Autodesk Inventor part; units mm, degrees
ref_plane "YZ Plane" through (0, 0, 0) normal (1, 0, 0) x (0, 1, 0)
ref_plane "XZ Plane" through (0, 0, 0) normal (0, 1, 0) x (-1, 0, 0)
ref_plane "XY Plane" through (0, 0, 0) normal (0, 0, 1) x (1, 0, 0)
sketch "Эскиз1" plane through (0, 0, 0) normal (0, 0, 1) x (1, 0, 0)
  line L0 (-19.4221, 3.2482) -> (-17.0252, 13.9839)
  line L1 (17.0252, 13.9839) -> (19.4221, 3.2482)
  arc A0 (-41.5809, 15.0397) -> (41.5809, 15.0397) centre (0, 65) ccw
  line L2 (41.5809, 15.0397) -> (33.2647, 25.0318)
  arc A1 (-33.2647, 25.0318) -> (33.2647, 25.0318) centre (0, 65) ccw
  line L3 (-33.2647, 25.0318) -> (-41.5809, 15.0397)
  line L4 (-5.5, 11.5) -> (-5.5, 0.5)
  line L5 (5.5, 0.5) -> (5.5, 11.5)
  circle A2 centre (0, 65) radius 65
  circle A3 centre (0, 65) radius 52
  line L6 (-41.5809, 15.0397) -> (-33.2647, 25.0318)
  line L7 (20.5764, 3.3428) -> (0, 65)
  line L8 (-41.5809, 15.0397) -> (0, 65)
  line L9 (0, 65) -> (21.1137, 3.5247)
  line L10 (-32.5, 8.7083) -> (0, 65)
  line L11 (0, 65) -> (32.5, 8.7083)
  line L12 (0, 65) -> (0, 0)
  arc A4 (-39.7976, 13.9446) -> (-45.7382, 14.0977) centre (-42.8715, 10.0011) ccw
  line L13 (-45.7382, 14.0977) -> (-66.813, -0.6503)
  line L14 (-66.813, -0.6503) -> (-66.8135, -2.4814)
  line L15 (-66.8135, -2.4814) -> (-61.8135, -2.4828)
  line L16 (-61.8135, -2.4828) -> (-61.8127, 0.4976)
  arc A5 (-61.386, 1.3167) -> (-61.8127, 0.4976) centre (-60.8127, 0.4974) ccw
  line L17 (-61.386, 1.3167) -> (-46.2094, 11.9372)
  arc A6 (-40.3216, 11.8247) -> (-46.2094, 11.9372) centre (-43.3426, 7.8406) ccw
  arc A7 (-40.3216, 11.8247) -> (-21.0718, 1.6801) centre (0, 65) ccw
  line L18 (-21.0718, 1.6801) -> (-20.6332, 3.6423)
  arc A8 (-39.7976, 13.9446) -> (-20.6332, 3.6423) centre (0, 65) ccw
  circle A9 centre (0, 65) radius 64.7341
  arc A10 (-42.6225, 16.2781) -> (-20.6332, 3.6423) centre (0, 65) ccw
  line L19 (-42.6225, 16.2781) -> (0, 65)
  point P0 (0, 0)
  point P1 (0, 13)
  point P2 (-26, 19.9667)
  point P3 (-32.5, 8.7083)
  point P4 (32.5, 8.7083)
  point P5 (26, 19.9667)
  dimension "d23" = 0.5
  dimension "d25" = 60
  dimension "d26" = 30
  dimension "d42" = 60.135
extrude "Выдавливание1" add sketch "Эскиз1" along normal blind 10 contours L7 A9 L1 | L7 A1 L9 A9 | L1 A9 L12 A1 L7 | A9 L7 A0 L12 | A9 L9 A0 L7 | A9 L11 A0 L9 | L9 A1 L11 A9 | L12 A9 A8 L10 A1 | L12 A0 L18 A9 | A0 L10 A8 L18
sketch "Эскиз4" plane through (0, 0, 10) normal (0, 0, 1) x (1, 0, 0)
  arc A0 (-13.3607, 13.1952) -> (-9.9415, 12.4318) centre (0, 65) ccw
  circle A1 centre (0, 65) radius 53.5
  circle A2 centre (0, 65) radius 54.5
  line L0 (-26, 19.9667) -> (-32.5, 8.7083)
  arc A3 (-26, 19.9667) -> (-22.4589, 18.1001) centre (0, 65) ccw
  arc A4 (-26, 19.9667) -> (26, 19.9667) centre (0, 65) ccw
  arc A5 (22.4589, 18.1001) -> (26, 19.9667) centre (0, 65) ccw
  line L1 (32.5, 8.7083) -> (26, 19.9667)
  point P0 (0, 0)
  point P1 (-27.25, 17.8016)
  point P2 (27.25, 17.8016)
  dimension "d43" = 1
extrude "Выдавливание4" cut sketch "Эскиз4" against normal blind 5 contours A1 L0 A3 A4 L1 A0 | A0 A1 L1 A2 L0
draft "НаклГрань1" angle 10 pull direction (0, 0, -1) faces at (-30.75, 11.7394, 5) fixed edges at (-26.625, 18.8841, 5)
draft "НаклГрань2" angle 10 pull direction (0, 0, -1) faces at (30.75, 11.7394, 5) fixed edges at (26.625, 18.8841, 5)
sketch "Эскиз5" plane through (0, 0, 10) normal (0, 0, 1) x (1, 0, 0)
  arc A0 (-26, 19.9667) -> (26, 19.9667) centre (0, 65) ccw
  line L0 (-27.25, 17.8016) -> (-26, 19.9667)
  arc A1 (-27.25, 17.8016) -> (27.25, 17.8016) centre (0, 65) ccw
  line L1 (26, 19.9667) -> (27.25, 17.8016)
  point P0 (0, 0)
extrude "Выдавливание5" cut sketch "Эскиз5" against normal blind 6
sketch "Эскиз6" plane through (0, 0, 0) normal (0, 0, -1) x (-1, 0, 0)
  line L0 (-31.7335, 8.2727) -> (-25.2327, 19.5323)
  arc A0 (-25.2327, 19.5323) -> (25.2327, 19.5323) centre (0, 65) ccw
  arc A1 (-31.7335, 8.2727) -> (31.7335, 8.2727) centre (0, 65) ccw
  line L1 (25.2327, 19.5323) -> (31.7335, 8.2727)
  circle A2 centre (0, 20) radius 1.925
  circle A3 centre (0, 20) radius 4
  circle A4 centre (0, 20) radius 1.6
  circle A5 centre (0, 20) radius 4
  line L2 (-2.8284, 22.8284) -> (-11.3933, 14.2635)
  line L3 (2.8284, 22.8284) -> (11.3933, 14.2635)
  line L4 (0, 89.6007) -> (0, 9.3033)
  point P0 (0, 0)
  dimension "d50" = 3.2
  dimension "d51" = 8
  dimension "d52" = 45
  dimension "d53" = 45
extrude "Выдавливание6" add sketch "Эскиз6" against normal blind 2.5 contours L2 A3 L4 A0 | L4 A3 L3 A0 | A3 L4 A2 | L4 A2 A3 | L4 A4 A2 | A2 L4 A4
equation "\"d26\" = 0.5 * d25"
properties part number "vzuh_karetka"
Geometry: final body of the model. Coordinates: model frame, mm. A direction names the side the tool comes from. Round coordinates to 2 decimals unless told otherwise and drop trailing zeros. Order: outer loops, then holes, each group sorted by start corner. A loop starts at its lowest first (then second) coordinate and runs counter-clockwise, first axis right, second up. Notation, with made-up numbers: M 31,-33 L 65,-33 A31 cw 65,-7 Z; hole C -16.5,3 d5. An arc over 180 degrees is marked long. Use one line per item in the form item = value. Start each with the question number.
Q1. Cut plane B-B (z = 1.5). Return loops of the section in (x, y).
Q2. Material intervals for line 1 (Y direction, x = 0, z = 1.55); line 2 (Z direction, x = 2, y = 12); line 3 (Z direction, x = -6, y = 18.75), sorted ascending. Write a range as [from, to].
Q3. Pin query (flat end, axial travel): pin 1 Ø7.5 at (x, y) = (-10.5, 17) entering from +Z; pin 2 Ø1 at (y, z) = (14, 5.5) entering from -X; pin 3 Ø1.5 at (y, z) = (4.5, 8) entering from -X. Return the tip coordinate at first contact, or that it passes through.
Q4. Access query for faces 1 (the face through (-7.051, 18.606, 1.232)), 2 (the face through (-0.1, 12.8, 4)), 3 (the face through (0, 0, 5)). Directions: +Z, -Z, +X, -X, +Y, -Y. A direction counts if a zero-diameter tool reaches every point of the face in a straight line with its end or side. Return the directions, or none.
Q5. Cut plane C-C (x = 12). Return loops of the section in (y, z).
Q6. Cut plane D-D (y = 3.25). Return loops of the section in (x, z).
Q7. Cut plane A-A (x = 0). Return loops of the section in (y, z).
Geometry results:
q1.outline = M -31.96,8.4 A65 ccw 31.96,8.4 L 25.46,19.66 A52 cw 11.39,14.26 L 2.83,22.83 A4 ccw -2.83,22.83 L -11.39,14.26 A52 cw -25.46,19.66 Z; hole C 0,20 d3.2
q2.line_1 = [0, 18.4], [21.6, 24]
q2.line_2 = [0, 4]
q2.line_3 = [0, 2.5]
q3.pin_1 = 4
q3.pin_2 = -29.85
q3.pin_3 = -25.59
q4.face_1 = +Z, -Z, +Y
q4.face_2 = +Z, +Y
q4.face_3 = +Z, -Z, -Y
q5.outline = M 1.12,0 L 14.4,0 L 14.4,4 L 11.84,4 L 11.84,10 L 1.12,10 Z
q6.outline = M -20.3,0 L 20.3,0 L 20.3,10 L -20.3,10 Z
q7.outline = M 0,0 L 18.4,0 L 18.4,2.5 L 13,2.5 L 13,4 L 10.5,4 L 10.5,10 L 0,10 Z; M 21.6,0 L 24,0 L 24,2.5 L 21.6,2.5 Z
